Here's how the part is built. I have some questions about the finished solid (model axes, mm). Face numbers are marked on the shaded views. A direction names the side the tool comes from. Give positions to 0.01 mm unless a question says otherwise; leave off trailing zeros. Order: outer loops, then holes, each group sorted by start corner. A loop starts at its lowest first (then second) coordinate and runs counter-clockwise, first axis right, second up.
from build123d import *

# Parameters (mm, degrees)
F1_DEPTH = 55
F2_R     = 4
F3_R     = 2.8
F4_DEPTH = 25


with BuildPart() as f1:
    # F0 (on Right) → F1 (new body)
    with BuildSketch(Plane.YZ):
        Polygon((-0.4503256133, 6.495247405), (-0.4503256133, -1.504752595), (79.5496743867, -1.2945870653), (79.5496743867, -0.2945870653), align=None)
    extrude(amount=F1_DEPTH)

    # F2
    f2_edges = [f1.edges().sort_by_distance(p)[0] for p in [
        (0, -0.450326, 2.495247),
        (55, -0.450326, 2.495247),
        (0, 79.549674, -0.794587),
        (55, 79.549674, -0.794587),
    ]]
    fillet(f2_edges, radius=F2_R)

    # F3 (on face) → F4 (cut)
    with BuildSketch(Plane(origin=(0, 0.5441073712, 6.4108469631), x_dir=(1, 0, 0), z_dir=(0, 0.0845688851, 0.9964176352))):
        with BuildLine():
            Line((10.5, 52.5083540007), (9.25, 52.5083540007))
            ThreePointArc((9.25, 52.5083540007), (5.7144660941, 51.0438879067), (4.25, 47.5083540007))
            Line((4.25, 47.5083540007), (4.25, 28.3626182626))
            ThreePointArc((4.25, 28.3626182626), (5.7144660941, 24.8270843567), (9.25, 23.3626182626))
            Line((9.25, 23.3626182626), (10.5, 23.3626182626))
            ThreePointArc((10.5, 23.3626182626), (14.0355339059, 24.8270843567), (15.5, 28.3626182626))
            Line((15.5, 28.3626182626), (15.5, 47.5083540007))
            ThreePointArc((15.5, 47.5083540007), (14.0355339059, 51.0438879067), (10.5, 52.5083540007))
        make_face()
        with BuildLine():
            Line((19.5, 29.0019917861), (35.5, 29.0019917861))
            ThreePointArc((35.5, 29.0019917861), (36.9142135624, 29.5877782237), (37.5, 31.0019917861))
            Line((37.5, 31.0019917861), (37.5, 47.0019917861))
            ThreePointArc((37.5, 47.0019917861), (36.9142135624, 48.4162053484), (35.5, 49.0019917861))
            Line((35.5, 49.0019917861), (19.5, 49.0019917861))
            ThreePointArc((19.5, 49.0019917861), (18.0857864376, 48.4162053484), (17.5, 47.0019917861))
            Line((17.5, 47.0019917861), (17.5, 31.0019917861))
            ThreePointArc((17.5, 31.0019917861), (18.0857864376, 29.5877782237), (19.5, 29.0019917861))
        make_face()
        with BuildLine():
            Line((50.75, 28.3626182626), (50.75, 47.5083540007))
            ThreePointArc((50.75, 47.5083540007), (49.2855339059, 51.0438879067), (45.75, 52.5083540007))
            Line((45.75, 52.5083540007), (44.5, 52.5083540007))
            ThreePointArc((44.5, 52.5083540007), (40.9644660941, 51.0438879067), (39.5, 47.5083540007))
            Line((39.5, 47.5083540007), (39.5, 28.3626182626))
            ThreePointArc((39.5, 28.3626182626), (40.9644660941, 24.8270843567), (44.5, 23.3626182626))
            Line((44.5, 23.3626182626), (45.75, 23.3626182626))
            ThreePointArc((45.75, 23.3626182626), (49.2855339059, 24.8270843567), (50.75, 28.3626182626))
        make_face()
        with BuildLine():
            ThreePointArc((22.5658532124, 3.7519917861), (23.9800667747, 4.3377782237), (24.5658532124, 5.7519917861))
            Line((24.5658532124, 5.7519917861), (24.5658532124, 23.3626182626))
            ThreePointArc((24.5658532124, 23.3626182626), (23.9800667747, 24.776831825), (22.5658532124, 25.3626182626))
            Line((22.5658532124, 25.3626182626), (19.6637449961, 25.3626182626))
            ThreePointArc((19.6637449961, 25.3626182626), (18.7013266797, 25.1158298826), (17.9764220206, 24.436369247))
            Line((17.9764220206, 24.436369247), (12.7626770245, 16.243341396))
            ThreePointArc((12.7626770245, 16.243341396), (12.5297596568, 15.7287657192), (12.45, 15.1695904116))
            Line((12.45, 15.1695904116), (12.45, 5.7519917861))
            ThreePointArc((12.45, 5.7519917861), (13.0357864376, 4.3377782237), (14.45, 3.7519917861))
            Line((14.45, 3.7519917861), (22.5658532124, 3.7519917861))
        make_face()
        with BuildLine():
            Line((30.4341467876, 23.3626182626), (30.4341467876, 5.7519917861))
            ThreePointArc((30.4341467876, 5.7519917861), (31.0199332253, 4.3377782237), (32.4341467876, 3.7519917861))
            Line((32.4341467876, 3.7519917861), (40.55, 3.7519917861))
            ThreePointArc((40.55, 3.7519917861), (41.9642135624, 4.3377782237), (42.55, 5.7519917861))
            Line((42.55, 5.7519917861), (42.55, 15.1695904116))
            ThreePointArc((42.55, 15.1695904116), (42.4702403432, 15.7287657192), (42.2373229755, 16.243341396))
            Line((42.2373229755, 16.243341396), (37.0235779794, 24.436369247))
            ThreePointArc((37.0235779794, 24.436369247), (36.2986733203, 25.1158298826), (35.3362550039, 25.3626182626))
            Line((35.3362550039, 25.3626182626), (32.4341467876, 25.3626182626))
            ThreePointArc((32.4341467876, 25.3626182626), (31.0199332253, 24.776831825), (30.4341467876, 23.3626182626))
        make_face()
        with BuildLine():
            ThreePointArc((32.4341467876, 74.2519917861), (31.0199332253, 73.6662053484), (30.4341467876, 72.2519917861))
            Line((30.4341467876, 72.2519917861), (30.4341467876, 54.6413653095))
            ThreePointArc((30.4341467876, 54.6413653095), (31.0199332253, 53.2271517471), (32.4341467876, 52.6413653095))
            Line((32.4341467876, 52.6413653095), (35.3362550039, 52.6413653095))
            ThreePointArc((35.3362550039, 52.6413653095), (36.2986733203, 52.8881536895), (37.0235779794, 53.5676143251))
            Line((37.0235779794, 53.5676143251), (42.2373229755, 61.7606421761))
            ThreePointArc((42.2373229755, 61.7606421761), (42.4702403432, 62.2752178529), (42.55, 62.8343931605))
            Line((42.55, 62.8343931605), (42.55, 72.2519917861))
            ThreePointArc((42.55, 72.2519917861), (41.9642135624, 73.6662053484), (40.55, 74.2519917861))
            Line((40.55, 74.2519917861), (32.4341467876, 74.2519917861))
        make_face()
        with BuildLine():
            Line((22.5658532124, 74.2519917861), (14.45, 74.2519917861))
            ThreePointArc((14.45, 74.2519917861), (13.0357864376, 73.6662053484), (12.45, 72.2519917861))
            Line((12.45, 72.2519917861), (12.45, 62.8343931605))
            ThreePointArc((12.45, 62.8343931605), (12.5297596568, 62.2752178529), (12.7626770245, 61.7606421761))
            Line((12.7626770245, 61.7606421761), (17.9764220206, 53.5676143251))
            ThreePointArc((17.9764220206, 53.5676143251), (18.7013266797, 52.8881536895), (19.6637449961, 52.6413653095))
            Line((19.6637449961, 52.6413653095), (22.5658532124, 52.6413653095))
            ThreePointArc((22.5658532124, 52.6413653095), (23.9800667747, 53.2271517471), (24.5658532124, 54.6413653095))
            Line((24.5658532124, 54.6413653095), (24.5658532124, 72.2519917861))
            ThreePointArc((24.5658532124, 72.2519917861), (23.9800667747, 73.6662053484), (22.5658532124, 74.2519917861))
        make_face()
        with Locations((48.2, 72.2019917861)):
            Circle(F3_R)
        with Locations((48.2, 5.8019917861)):
            Circle(F3_R)
        with Locations((6.8, 5.8019917861)):
            Circle(F3_R)
        with Locations((6.8, 72.2019917861)):
            Circle(F3_R)
    extrude(amount=-F4_DEPTH, mode=Mode.SUBTRACT)


solid = f1.part
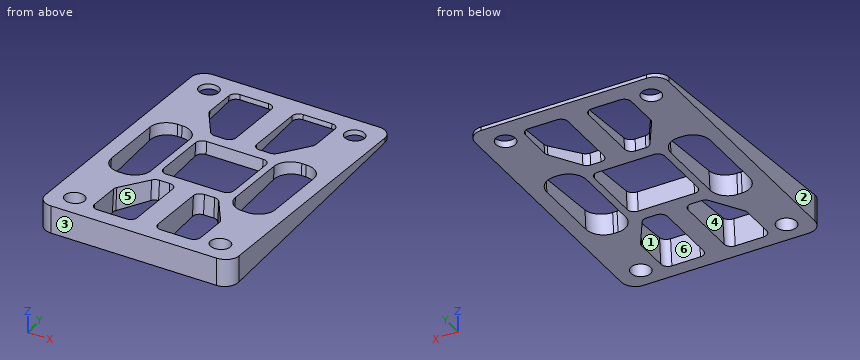
Q1. I'm going to push flat-ended pins straight in: P1, Ø12, axis at x = 34.5, y = 9, coming from the -Z side; P2, Ø1, axis at x = 11.5, z = 3, coming from the +Y side. Where does each tip first touch, or does it pass through?
Filled sheet:
P1: stops at z = -1.5
P2: stops at y = 23.94
Q2. I need wall thicknesses on L1, parallel to X at y = 43, z = 0.5; L2, parallel to X at y = 15, z = 4.5; L3, parallel to Y at x = 34, z = 0.75. Which ranges of each line are inside material? Lowest first, please.
Filled sheet:
L1: x = 0 to 4.25, 15.5 to 17.5, 37.5 to 39.5, 50.75 to 55
L2: x = 0 to 12.45, 24.57 to 30.43, 42.55 to 55
L3: y = -0.45 to 3.83, 25.52 to 29.17, 49.24 to 52.89
Q3. If we section it at A-A on y = 64: List the corners of the cut face in (x, z) for me, plus the area to 3 significant figures.
Filled sheet:
outline: (0, -1.34) - (12.45, -1.34) - (12.45, 1.03) - (0, 1.03) - close; (24.57, -1.34) - (30.43, -1.34) - (30.43, 1.03) - (24.57, 1.03) - close; (42.55, -1.34) - (55, -1.34) - (55, 1.03) - (42.55, 1.03) - close
area: 72.6 mm2
Q4. Thinking about a two-plate mould opening in Y: for the marked faces 1, 2 and 3, which applies, released by +Y, released by -Y, zero draft, split by the parting line, or undercut?
Filled sheet:
face 1: undercut
face 2: zero draft
face 3: released by -Y
Q5. For the marked faces 4, 5 and 6, which set-ups out of +Z, -Z, +X, -X, +Y, -Y let a thin tool reach every point of the face, with its end or its side?
Filled sheet:
face 4: +Z, -Z
face 5: +Z
face 6: -Z
Q6. If we section it at B-B on x = 47: List the corners of the cut face in (y, z) for me.
Filled sheet:
outline: (-0.45, -1.5) - (3.16, -1.5) - (3.8, 6.13) - (-0.45, 6.5) - close; (8.24, -1.48) - (23.48, -1.44) - (23.98, 4.42) - (8.85, 5.71) - close; (52.42, -1.37) - (69.81, -1.32) - (69.97, 0.52) - (52.71, 1.98) - close; (74.89, -1.31) - (79.55, -1.29) - (79.55, -0.29) - (75.01, 0.09) - close
